Can you work these out from the model? Positions are in its coordinate system, mm. Face numbers are marked on the shaded views. A direction names the side the tool comes from. Give positions to 0.01 mm unless a question says otherwise; leave off trailing zeros. Order: outer loops, then holes, each group sorted by start corner. A loop starts at its lowest first (then second) coordinate and runs counter-clockwise, first axis right, second up. Notation, with made-up numbers: (7.5, -0.5) - (59.5, -0.5) arc R26 cw to (59.5, 38.5) - close; hole circle Ø3 at (15.5, 61.25). An arc over 180 degrees is marked (long way). Return JSON: item names as keys, results as strings.
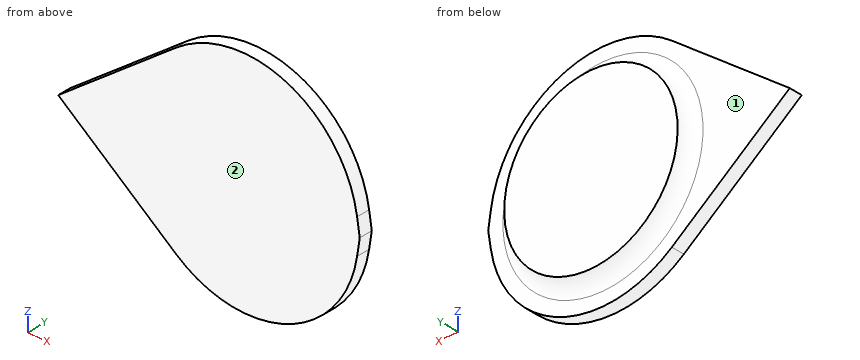
```python
from build123d import *

# Parameters (mm, degrees)
BOSS_EXTRUDE1_DEPTH = 5
SKETCH2_R           = 32.5
BOSS_EXTRUDE2_DEPTH = 5
FILLET1_R           = 5


with BuildPart() as part:
    # Sketch1 → Boss-Extrude1 (new body)
    with BuildSketch(Plane(origin=(0, 0, 0), x_dir=(1, 0, 0), z_dir=(0, 1, 0))):
        with BuildLine():
            Line((-25.803571429, 33.770189539), (-70, 0))
            Line((-70, 0), (-25.803571429, -33.770189539))
            ThreePointArc((-25.803571429, -33.770189539), (15.876337275, -39.423240794), (42.005813953, -6.462321108))
            Line((42.005813953, -6.462321108), (43, 0))
            Line((43, 0), (42.005813953, 6.462321108))
            ThreePointArc((42.005813953, 6.462321108), (15.876337275, 39.423240794), (-25.803571429, 33.770189539))
        make_face()
    extrude(amount=BOSS_EXTRUDE1_DEPTH)

    # Sketch2 → Boss-Extrude2 (add)
    with BuildSketch(Plane(origin=(0, 5, 0), x_dir=(1, 0, 0), z_dir=(0, 1, 0))):
        with Locations(Location((0, 0, 0), (0, 0, 270))):
            Circle(SKETCH2_R)
    extrude(amount=BOSS_EXTRUDE2_DEPTH)

    # Fillet1
    fillet1_edges = [part.edges().sort_by_distance(p)[0] for p in [
        (0, 5, -32.5),
    ]]
    fillet(fillet1_edges, radius=FILLET1_R - 0.0001)  # a hair under: the kernel refuses the full size


solid = part.part
```
1. On a 3-axis mill with a long thin cutter (end or side, diameter ignored), from which of +Z, -Z, +X, -X, +Y, -Y can I reach the whole of each face in a straight line? I mean the marked faces 1 and 2. Say none if no direction works.
Checks:
{"face 1": "+Y", "face 2": "+Z, -Z, +X, -X, -Y"}
2. Suppose I cut it at B-B (y = 2.5). List the corners of the cut face in (x, z) for me, plus the area to 3 significant figures.
Checks:
{"outline": "(-70, 0) - (-25.8, -33.77) arc R42.5 ccw to (42.01, -6.46) - (43, 0) - (42.01, 6.46) arc R42.5 ccw to (-25.8, 33.77) - close", "area": "6,380 mm^2"}
3. Suppose I cut it at C-C (x = -45). List the corners of the cut face in (y, z) for me.
Checks:
{"outline": "(0, -19.1) - (5, -19.1) - (5, 19.1) - (0, 19.1) - close"}
4. If I drill on L1, parallel to Y at x = -39.5, z = -4; L2, parallel to X at y = 9.75, z = -1; L3, parallel to X at y = 9, z = 20, over which ranges is the centre line in solid material (lowest first)? Write a range as [from, to].
Checks:
{"L1": "[0, 5]", "L2": "[-32.49, 32.49]", "L3": "[-25.75, 25.75]"}
5. For pin 1 Ø12 at (x, z) = (-14.5, 33) entering from +Y; pin 2 Ø5 at (y, z) = (1, -30.5) entering from +X; pin 3 Ø2 at (y, z) = (4, 12) entering from -X; pin 4 Ø1 at (y, z) = (8.5, 15) entering from -X, each with a flat end and sliding along its axis, tell me the tip position at first contact or that it passes through.
Checks:
{"pin 1": "y = 10", "pin 2": "x = 31.97", "pin 3": "x = -55.6", "pin 4": "x = -29.41"}
